The drawing under review shows one solid part. Ordinate dimensions are in mm from its lowest x, y, z. A direction names the side the tool comes from. Round coordinates to 2 decimals unless told otherwise and drop trailing zeros. Write each loop counter-clockwise with the first axis right and the second up, starting at its lowest first coordinate (ties: lowest second). Pieces come first, ordered by that corner, then holes.
Item 1: Add section C-C (z = 32). Give the boundary of the cut face in (x, y), plus the area to 3 significant figures.
Item 2: Draft analysis for pull direction Z (two halves, no side actions). For the marked faces 1, 2, 3 and 4, state which applies: +Z half, -Z half, draft (parallel to the pull), parting line (faces both ways), or undercut.
Item 3: To check wall thickness, follow L1, parallel to Z at x = 21, y = 2; L2, parallel to Y at x = 30, z = 6; L3, parallel to Z at x = 28.5, y = 35.5. State the ranges of each line that lie inside material, in increasing order.
Item 4: Machinability: for the marked faces 5, 6, 7, 8 and 9, which of the approach directions +Z, -Z, +X, -X, +Y, -Y give a long, thin tool a straight path to every point of the face, cutting with its end or side? Answer none if there is none.
Item 5: Add section A-A (y = 27.5). Give the boundary of the cut face in (x, z).
Item 6: Add section D-D (y = 18.5). Give the boundary of the cut face in (x, z), plus the area to 3 significant figures.
Item 7: Clearance check with flat-ended pins moving along their axes: pin 1 Ø3 at (y, z) = (27, 17) entering from -X; pin 2 Ø3 at (x, z) = (43, 10) entering from +Y; pin 3 Ø3 at (y, z) = (13, 26.5) entering from +X; pin 4 Ø8 at (x, y) = (41.5, 27) entering from +Z. State where each tip first meets the part, or that it passes through.
Item 8: Add section B-B (x = 38.5). Give the boundary of the cut face in (y, z), plus the area to 3 significant figures.
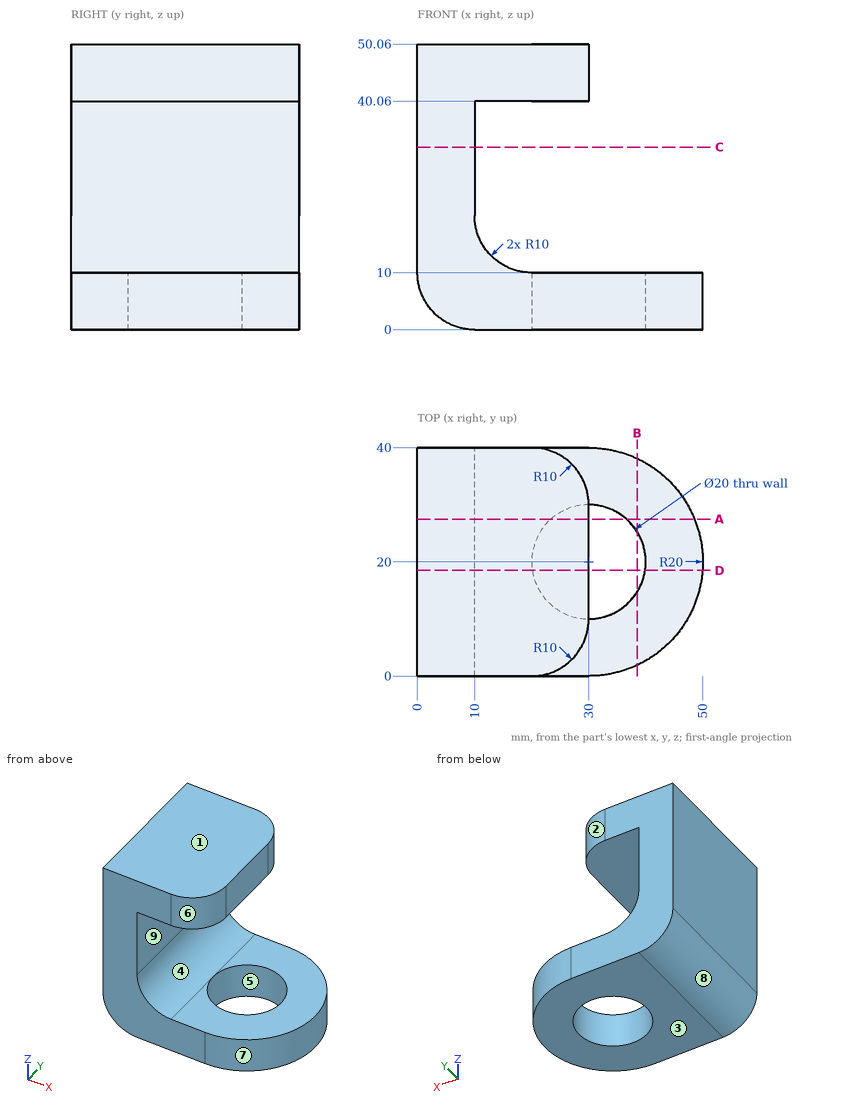
Numbers:
1. outline: (0, 0) - (10, 0) - (10, 40) - (0, 40) - close
1. area: 400 mm2
2. face 1: +Z half
2. face 2: draft
2. face 3: -Z half
2. face 4: undercut
3. L1: z = 0 to 10, 40.06 to 50.06
3. L2: y = 0 to 10, 30 to 40
3. L3: z = 0 to 10
4. face 5: -Z
4. face 6: +Z, +X, -Y
4. face 7: +Z, -Z, +X
4. face 8: -Z, -X, +Y, -Y
4. face 9: +X, +Y, -Y
5. outline: (0, 10) arc R10 ccw to (10, 0) - (23.39, 0) - (23.39, 10) - (20, 10) arc R10 cw to (10, 20) - (10, 40.06) - (30, 40.06) - (30, 50.06) - (0, 50.06) - close; (36.61, 0) - (48.54, 0) - (48.54, 10) - (36.61, 10) - close
6. outline: (0, 10) arc R10 ccw to (10, 0) - (20.11, 0) - (20.11, 10) - (20, 10) arc R10 cw to (10, 20) - (10, 40.06) - (30, 40.06) - (30, 50.06) - (0, 50.06) - close; (39.89, 0) - (49.94, 0) - (49.94, 10) - (39.89, 10) - close
6. area: 902 mm2
7. pin 1: stops at x = 0
7. pin 2: stops at y = 36.36
7. pin 3: stops at x = 10
7. pin 4: stops at z = 10
8. outline: (1.9, 0) - (14.73, 0) - (14.73, 10) - (1.9, 10) - close; (25.27, 0) - (38.1, 0) - (38.1, 10) - (25.27, 10) - close
8. area: 257 mm2
